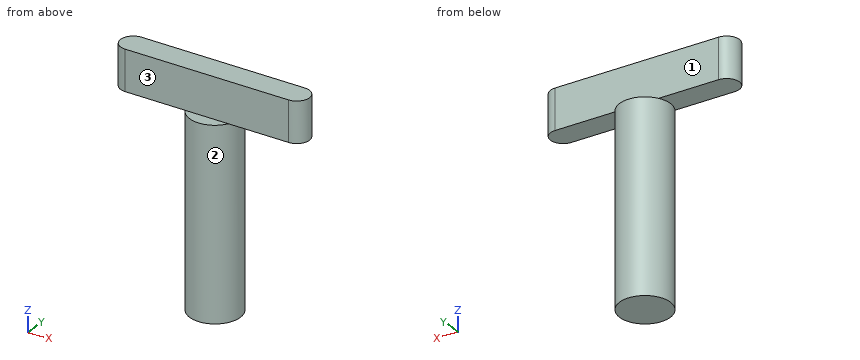
from build123d import *

# Parameters (mm, degrees)
F1_DEPTH = 6.42
F2_R     = 4
F3_DEPTH = 30


with BuildPart() as f1:
    # F0 (on Top) → F1 (new body)
    with BuildSketch(Plane.XY):
        with BuildLine():
            Line((13, 2), (-13, 2))
            ThreePointArc((-13, 2), (-15, 0), (-13, -2))
            Line((-13, -2), (13, -2))
            ThreePointArc((13, -2), (15, 0), (13, 2))
        make_face()
    extrude(amount=F1_DEPTH)

    # F2 (on face) → F3 (join)
    with BuildSketch(Plane(origin=(0, 0, 0), x_dir=(1, 0, 0), z_dir=(0, 0, -1))):
        Circle(F2_R)
    extrude(amount=F3_DEPTH)


solid = f1.part
The listing builds one solid part. Answer for the finished solid, in the listing's coordinates (mm). Face numbers are marked on the shaded views. A direction names the side the tool comes from. Round coordinates to 2 decimals unless told otherwise and drop trailing zeros. Order: outer loops, then holes, each group sorted by start corner. A loop starts at its lowest first (then second) coordinate and runs counter-clockwise, first axis right, second up. Notation, with made-up numbers: (28, 79.5) - (62, 79.5) arc R27 ccw to (62, 106.5) - close; hole circle Ø4 at (82.25, 30). An arc over 180 degrees is marked (long way). Write item = value, one per line. Start each with the question number.
1) Section C-C, the plane z = -6 is taken. Write down the section's boundary in (x, y), plus the area to 3 significant figures.
2) For the marked faces 1, 2 and 3, determine the directions among +Z, -Z, +X, -X, +Y, -Y from which every point of the face is accessible in a straight line to the end or side of a thin tool.
3) Section D-D, the plane z = 4 is taken. Write down the section's boundary in (x, y).
4) Given pin 1 (0.6 mm diameter, centred on x = -1, y = 3, fed in from +Z); pin 2 (7 mm diameter, centred on x = -2.5, z = 4.5, fed in from -Y); pin 3 (1 mm diameter, centred on y = 2, z = -11, fed in from -X), each flat-ended and moving along its own axis, determine where each tip first touches the part or whether it passes through.
5) Straight lines are drawn through the part: L1, parallel to Z at x = -5.5, y = -0.25; L2, parallel to X at y = -0.25, z = -18; L3, parallel to Y at x = 2, z = -9. For each, find the intervals that lie inside material, in ascending order.
6) Section A-A, the plane y = 0 is taken. Write down the section's boundary in (x, z), plus the area to 3 significant figures.
7) Section B-B, the plane x = 0 is taken. Write down the section's boundary in (y, z), plus the area to 3 significant figures.
Results list:
q1.outline = circle Ø8 at (0, 0)
q1.area = 50.3 mm^2
q2.face_1 = +Z, +X, -X, +Y
q2.face_2 = -Z
q2.face_3 = +Z, +X, -X, -Y
q3.outline = (-13, -2) - (13, -2) arc R2 ccw to (13, 2) - (-13, 2) arc R2 ccw to start
q4.pin_1 = 0
q4.pin_2 = -2
q4.pin_3 = -3.71
q5.L1 = 0 to 6.42
q5.L2 = -3.99 to 3.99
q5.L3 = -3.46 to 3.46
q6.outline = (-15, 0) - (-4, 0) - (-4, -30) - (4, -30) - (4, 0) - (15, 0) - (15, 6.42) - (-15, 6.42) - close
q6.area = 433 mm^2
q7.outline = (-4, -30) - (4, -30) - (4, 0) - (2, 0) - (2, 6.42) - (-2, 6.42) - (-2, 0) - (-4, 0) - close
q7.area = 266 mm^2
